Work out the finished part from the listing and answer in its coordinate system (mm). A direction names the side the tool comes from. Round coordinates to 2 decimals unless told otherwise and drop trailing zeros. Loops run counter-clockwise (first coordinate to the right, second up) from the corner with the lowest first, then second, coordinate; pieces in that order, holes last. Notation, with made-up numbers: (15.5, -12.5) - (53.5, -12.5) arc R20 cw to (53.5, -2.5) - close; hole circle Ø7 at (34, 80). An arc over 180 degrees is marked (long way). Use CSV: the item, a comma, the result in double quotes. Start each with the question number.
from build123d import *

# Parameters (mm, degrees)
F1_DEPTH = 25.4


with BuildPart() as f1:
    # F0 (on Front) → F1 (new body)
    with BuildSketch(Plane.XZ):
        with BuildLine():
            ThreePointArc((-23.4881200852, 9.1129863922), (-25.7569087098, 4.6952436795), (-27.3750988376, 0))
            ThreePointArc((-27.3750988376, 0), (-23.4523587377, -26.5236540337), (-1.822285639, -42.3676450379))
            add(Edge.make_bspline(
                [(31.6214489009, -32.408137431), (24.0381488742, -39.1257279454), (12.1793845571, -42.1949100042), (-1.822285639, -42.3676450379)],
                knots=[0.3305657958, 0.3305657958, 0.3305657958, 0.3305657958, 0.4117411776, 0.4117411776, 0.4117411776, 0.4117411776], degree=3))
            ThreePointArc((31.6214489009, -32.408137431), (39.9732334064, -17.2802023076), (40.0097537836, 0))
            Line((40.0097537836, 0), (24.3855283995, 0))
            Line((24.3855283995, 0), (24.3855283995, 20.8383404807))
            ThreePointArc((24.3855283995, 20.8383404808), (0.9049170427, 25.4619632407), (-20.0263610495, 13.8602998023))
            ThreePointArc((-20.0263610495, 13.8602998023), (-21.7035792641, 11.4475130703), (-23.4881200852, 9.1129863922))
        make_face()
        with BuildLine():
            ThreePointArc((-1.822285639, -42.3676450379), (-23.4523587377, -26.5236540337), (-27.3750988376, 0))
            ThreePointArc((-27.3750988376, 0), (-25.7569087098, 4.6952436795), (-23.4881200852, 9.1129863922))
            ThreePointArc((-23.4881200852, 9.1129863922), (-62.2831037982, -14.1508466737), (-106.8623494937, -6.4731163171))
            add(Edge.make_bspline(
                [(-1.822285639, -42.3676450379), (-34.1627739251, -42.7666213928), (-77.9356396487, -27.7130872373), (-106.8623494937, -6.4731163171)],
                knots=[0.4117411776, 0.4117411776, 0.4117411776, 0.4117411776, 0.5992367726, 0.5992367726, 0.5992367726, 0.5992367726], degree=3))
        make_face()
        with BuildLine():
            add(Edge.make_bspline(
                [(31.6214489009, -32.408137431), (24.0381488742, -39.1257279454), (12.1793845571, -42.1949100042), (-1.822285639, -42.3676450379)],
                knots=[0.3305657958, 0.3305657958, 0.3305657958, 0.3305657958, 0.4117411776, 0.4117411776, 0.4117411776, 0.4117411776], degree=3))
            ThreePointArc((-1.822285639, -42.3676450379), (2.2189423584, -43.0915267187), (6.317327473, -43.3339475664))
            Line((6.317327473, -43.3339475664), (21.2019422511, -39.9863561607))
            ThreePointArc((21.2019422511, -39.9863561607), (26.7658232425, -36.6841469116), (31.6214489009, -32.408137431))
        make_face()
        with BuildLine():
            ThreePointArc((-106.8623494937, -6.4731163171), (-62.2831037982, -14.1508466737), (-23.4881200852, 9.1129863922))
            ThreePointArc((-23.4881200852, 9.1129863922), (-21.8574061869, 11.5596842489), (-20.0263610495, 13.8602998023))
            ThreePointArc((-20.0263610495, 13.8602998023), (-11.9815447312, 31.0090830109), (-9.2218346427, 49.7489825666))
            ThreePointArc((-9.2218346427, 49.7489825666), (-15.373040222, 77.3515736193), (-32.6625531747, 99.7304275837))
            add(Edge.make_bspline(
                [(-136.0971185339, 29.794675775), (-147.1795152867, 70.6622045283), (-83.4949169934, 115.3318185014), (-32.6625531747, 99.7304275837)],
                knots=[0.6952883419, 0.6952883419, 0.6952883419, 0.6952883419, 1, 1, 1, 1], degree=3))
            ThreePointArc((-136.0971185339, 29.794675775), (-134.3309912676, 24.9782257744), (-132.1905665466, 20.3160397911))
            add(Edge.make_bspline(
                [(-106.8623494937, -6.4731163171), (-118.0127633165, 1.7142809574), (-126.9572157407, 10.8209088266), (-132.1905665466, 20.3160397911)],
                knots=[0.5992367726, 0.5992367726, 0.5992367726, 0.5992367726, 0.6715109264, 0.6715109264, 0.6715109264, 0.6715109264], degree=3))
        make_face()
        with BuildLine():
            ThreePointArc((-34.7453205512, 50.2754222832), (-74.1782043044, 18.8325014661), (-113.1855020537, 50.8018666913))
            Line((-113.1855020537, 50.8018666913), (-101.7999106632, 50.7254532919))
            ThreePointArc((-101.7999106632, 50.7254532918), (-78.0602804594, 87.7213526899), (-44.8327322387, 58.9429466583))
            ThreePointArc((-44.8327322387, 58.9429466583), (-45.1591089284, 54.5986268514), (-46.1309119417, 50.3518356826))
            Line((-46.1309119417, 50.3518356826), (-34.7453205512, 50.2754222832))
        make_face(mode=Mode.SUBTRACT)
        with BuildLine():
            Line((21.2019422511, -39.9863561607), (6.317327473, -43.3339475664))
            ThreePointArc((6.317327473, -43.3339475664), (13.9455337712, -42.486726351), (21.2019422511, -39.9863561607))
        make_face()
        with BuildLine():
            add(Edge.make_bspline(
                [(42.2519440934, 0), (43.0667519502, -13.4532818738), (39.8786763522, -25.0935550451), (31.6214489009, -32.408137431)],
                knots=[0.2421763625, 0.2421763625, 0.2421763625, 0.2421763625, 0.3305657958, 0.3305657958, 0.3305657958, 0.3305657958], degree=3))
            ThreePointArc((31.6214489009, -32.408137431), (26.7658232425, -36.6841469116), (21.2019422511, -39.9863561607))
            Line((21.2019422511, -39.9863561607), (198.9958948854, 0))
            Line((198.9958948854, 0), (162.1864286042, 0))
            ThreePointArc((162.1864286042, 0), (154.7074790766, -3.9710732295), (146.3514873037, -5.3427547241))
            Line((146.3514873037, -5.3427547241), (146.3514873037, -7.1069937982))
            Line((146.3514873037, -7.1069937982), (47.9064245235, -7.1069937982))
            Line((47.9064245235, -7.1069937982), (47.9064245235, 0))
            Line((47.9064245235, 0), (42.2519440934, 0))
        make_face()
        with BuildLine():
            ThreePointArc((-132.1905665466, 20.3160397911), (-121.4653525437, 5.0883042782), (-106.8623494937, -6.4731163171))
            add(Edge.make_bspline(
                [(-106.8623494937, -6.4731163171), (-118.0127633165, 1.7142809574), (-126.9572157407, 10.8209088266), (-132.1905665466, 20.3160397911)],
                knots=[0.5992367726, 0.5992367726, 0.5992367726, 0.5992367726, 0.6715109264, 0.6715109264, 0.6715109264, 0.6715109264], degree=3))
        make_face()
        with BuildLine():
            ThreePointArc((-9.2218346427, 49.7489825666), (-11.9815447312, 31.0090830109), (-20.0263610495, 13.8602998023))
            ThreePointArc((-20.0263610495, 13.8602998023), (0.9049170427, 25.4619632407), (24.3855283995, 20.8383404808))
            Line((24.3855283995, 20.8383404807), (24.3855283995, 51.0906824548))
            add(Edge.make_bspline(
                [(-15.5554291457, 92.0261433749), (0.3390335994, 82.5415688484), (14.2065732282, 67.591169523), (24.3855283995, 51.0906824548)],
                knots=[0.0353561549, 0.0353561549, 0.0353561549, 0.0353561549, 0.1378329831, 0.1378329831, 0.1378329831, 0.1378329831], degree=3))
            Line((-15.5554291457, 92.0261433749), (-23.7091819765, 96.3155100856))
            add(Edge.make_bspline(
                [(-32.6625531747, 99.7304275837), (-29.6292369493, 98.7994468334), (-26.6416857173, 97.653849539), (-23.7091819765, 96.3155100856)],
                knots=[0, 0, 0, 0, 0.0181830383, 0.0181830383, 0.0181830383, 0.0181830383], degree=3))
            ThreePointArc((-32.6625531747, 99.7304275837), (-15.373040222, 77.3515736193), (-9.2218346427, 49.7489825666))
        make_face()
        with BuildLine():
            Line((24.3855283995, 0), (40.0097537836, 0))
            ThreePointArc((40.0097537836, 0), (34.2162475505, 11.9326862666), (24.3855283995, 20.8383404808))
            Line((24.3855283995, 20.8383404807), (24.3855283995, 0))
        make_face()
        with BuildLine():
            ThreePointArc((24.3855283995, 20.8383404808), (34.2162475505, 11.9326862666), (40.0097537836, 0))
            Line((40.0097537836, 0), (42.2519440934, 0))
            add(Edge.make_bspline(
                [(24.3855283995, 51.0906824548), (34.7498868563, 34.2896493617), (41.2900666127, 15.8815465109), (42.2519440934, 0)],
                knots=[0.1378329831, 0.1378329831, 0.1378329831, 0.1378329831, 0.2421763625, 0.2421763625, 0.2421763625, 0.2421763625], degree=3))
            Line((24.3855283995, 51.0906824548), (24.3855283995, 20.8383404807))
        make_face()
        with BuildLine():
            add(Edge.make_bspline(
                [(24.3855283995, 51.0906824548), (34.7498868563, 34.2896493617), (41.2900666127, 15.8815465109), (42.2519440934, 0)],
                knots=[0.1378329831, 0.1378329831, 0.1378329831, 0.1378329831, 0.2421763625, 0.2421763625, 0.2421763625, 0.2421763625], degree=3))
            Line((42.2519440934, 0), (47.9064245235, 0))
            Line((47.9064245235, 0), (47.9064245235, 20.7945478899))
            Line((47.9064245235, 20.7945478899), (120.2141846897, 20.7945478899))
            ThreePointArc((120.2141846897, 20.7945478899), (146.3514873037, 46.931850504), (172.4887899177, 20.7945478899))
            ThreePointArc((172.4887899177, 20.7945478899), (169.7720043836, 9.1911877022), (162.1864286042, 0))
            Line((162.1864286042, 0), (198.9958948854, 0))
            Line((198.9958948854, 0), (198.9958948854, 51.0906824548))
            Line((198.9958948854, 51.0906824548), (24.3855283995, 51.0906824548))
        make_face()
        with BuildLine():
            add(Edge.make_bspline(
                [(-132.1905665466, 20.3160397911), (-133.9122824029, 23.4398352609), (-135.2323312991, 26.6056799314), (-136.0971185339, 29.794675775)],
                knots=[0.6715109264, 0.6715109264, 0.6715109264, 0.6715109264, 0.6952883419, 0.6952883419, 0.6952883419, 0.6952883419], degree=3))
            ThreePointArc((-132.1905665466, 20.3160397911), (-134.3309912676, 24.9782257744), (-136.0971185339, 29.794675775))
        make_face()
        with BuildLine():
            ThreePointArc((-49.373536191, 109.8165112697), (-118.3123179762, 97.5246309308), (-136.0971185339, 29.794675775))
            add(Edge.make_bspline(
                [(-136.0971185339, 29.794675775), (-147.1795152867, 70.6622045283), (-83.4949169934, 115.3318185014), (-32.6625531747, 99.7304275837)],
                knots=[0.6952883419, 0.6952883419, 0.6952883419, 0.6952883419, 1, 1, 1, 1], degree=3))
            ThreePointArc((-32.6625531747, 99.7304275837), (-35.6692605933, 102.0849992123), (-38.8090434498, 104.2589496877))
            Line((-38.8090434498, 104.2589496877), (-49.373536191, 109.8165112697))
        make_face()
        with BuildLine():
            ThreePointArc((-38.8090434498, 104.2589496877), (-35.6692605933, 102.0849992123), (-32.6625531747, 99.7304275837))
            add(Edge.make_bspline(
                [(-32.6625531747, 99.7304275837), (-29.6292369493, 98.7994468334), (-26.6416857173, 97.653849539), (-23.7091819765, 96.3155100856)],
                knots=[0, 0, 0, 0, 0.0181830383, 0.0181830383, 0.0181830383, 0.0181830383], degree=3))
            Line((-23.7091819765, 96.3155100856), (-38.8090434498, 104.2589496877))
        make_face()
        with BuildLine():
            Line((-23.7091819765, 96.3155100856), (-15.5554291457, 92.0261433749))
            add(Edge.make_bspline(
                [(-23.7091819765, 96.3155100856), (-20.9395552466, 95.0515046312), (-18.2190309331, 93.615572981), (-15.5554291457, 92.0261433749)],
                knots=[0.0181830383, 0.0181830383, 0.0181830383, 0.0181830383, 0.0353561549, 0.0353561549, 0.0353561549, 0.0353561549], degree=3))
        make_face()
        with BuildLine():
            ThreePointArc((-38.8090434498, 104.2589496877), (-43.9634537245, 107.2807369641), (-49.373536191, 109.8165112697))
            Line((-49.373536191, 109.8165112697), (-38.8090434498, 104.2589496877))
        make_face()
    extrude(amount=F1_DEPTH)


solid = f1.part
Item 1: Find the intervals of material crossed by probe 1 along X at (y, z) = (-8.25, 7.5); probe 2 along X at (y, z) = (-6, 51); probe 3 along Z at (x, y) = (88, -0.75), in increasing order. Write a range as [from, to].
Item 2: A cutting plane is placed at B-B (y = -12.75). State how many separate pieces and enclosed holes the cut face has, plus the area to 3 significant figures.
Item 3: Each of these flat-tipped pins is pushed along its axis until it touches: pin 1 Ø4 at (y, z) = (-3.5, 19.5) entering from -X; pin 2 Ø1 at (x, y) = (-58.5, -15) entering from -Z; pin 3 Ø1.8 at (x, y) = (41, -17) entering from -Z. Where does it stop, or does it pass through?
Item 4: A cutting plane is placed at A-A (x = 99). Determine the outline of the cut face in (y, z).
Item 5: The mould has two halves that part along Z. Classify faces 1 (the flat face through (108.854, -12.522, -20.273)), 2 (the flat face through (-10, 0, 19)), 3 (the flat face through (84, -13, 20.795)), 4 (the flat face through (47.906, -13, 7)): pulls with the +Z half, pulls with the -Z half, needs draft (parallel to the pull), parting line crosses it, or undercut.
Item 6: Which of the six approach directions +Z, -Z, +X, -X, +Y, -Y give full straight-line access (tool end or side, diameter ignored) to faces 5 (the flat face through (198.996, -13, 25)), 6 (the flat face through (113, -13, 51.091)), 7 (the flat face through (98, -13, -7.107))?
Item 7: A cutting plane is placed at D-D (x = 133.5). Determine the outline of the cut face in (y, z), plus the area to 3 significant figures.
Result sheet:
1,probe 1,"[-123.63, 47.91], [168.86, 199]"
1,probe 2,"[-139.22, -101.88], [-45.94, 199]"
1,probe 3,"[-24.96, -7.11], [20.79, 51.09]"
2,separate pieces,"1"
2,enclosed holes,"4"
2,area,"24,000 mm^2"
3,pin 1,"x = -132.82"
3,pin 2,"z = -31.71"
3,pin 3,"z = -35.74"
4,outline,"(-25.4, -22.49) - (0, -22.49) - (0, -7.11) - (-25.4, -7.11) - close; (-25.4, 20.79) - (0, 20.79) - (0, 51.09) - (-25.4, 51.09) - close"
5,face 1,"pulls with the -Z half"
5,face 2,"needs draft"
5,face 3,"undercut"
5,face 4,"undercut"
6,face 5,"+Z, -Z, +X, +Y, -Y"
6,face 6,"+Z, +X, +Y, -Y"
6,face 7,"+Y, -Y"
7,outline,"(-25.4, -14.73) - (0, -14.73) - (0, -7.11) - (-25.4, -7.11) - close; (-25.4, 43.55) - (0, 43.55) - (0, 51.09) - (-25.4, 51.09) - close"
7,area,"385 mm^2"
